Check sheet for the modelled part. Datum: model origin and axes. Units: mm. A direction names the side the tool comes from. Round coordinates to 2 decimals unless told otherwise and drop trailing zeros. Write each loop counter-clockwise with the first axis right and the second up, starting at its lowest first coordinate (ties: lowest second). Pieces come first, ordered by that corner, then holes.
Item 1: Go/stop test with flat-tipped pins: pin 1 Ø0.5 at (x, z) = (5, 3.5) entering from -Y; pin 2 Ø0.8 at (x, z) = (6, 3.5) entering from +Y; pin 3 Ø1.1 at (x, y) = (8.5, -21.5) entering from +Z. Record where each tip stops, or that it passes through.
Item 2: Cross-section at D-D on x = 6.35. Enter the section's corners in (y, z) (3 decimals).
Item 3: Cross-section at B-B on x = 11.5. Enter the section's corners in (y, z) (3 decimals), plus the area to 3 significant figures.
Item 4: Tool access check on faces 1 (the flat face through (6, -20.32, 3)), 2 (the flat face through (6, -6, 2.54)), 3 (the cylindrical face through (6.439, -25.038, 0.382)). Record the directions out of +Z, -Z, +X, -X, +Y, -Y that give a thin tool (end or side, any length) a straight path to the whole face; none if there is none.
Item 5: Cross-section at A-A on y = -6.35. Enter the section's corners in (x, z), plus the area to 3 significant figures.
Item 6: Release check for a two-part mould opening along Y. For faces 4 (the flat face through (6, -21, 1.778)), 5 (the flat face through (6, -23, 3.81)), 6 (the flat face through (6, -25.4, 2)) record: +Y half, -Y half, draft (parallel to the pull), parting line (faces both ways), or undercut.
Item 7: Cross-section at C-C on z = 0.5. Enter the section's corners in (x, y).
Item 8: Material ranges on line 1 (X direction, y = -6.35, z = 3.2); line 2 (Y direction, x = 6, z = 3.05); line 3 (Y direction, x = 6.35, z = 3.25), recorded low to high.
from build123d import *

# Parameters (mm, degrees)
F0_W        = 12.7
F0_H        = 25.4
F1_DEPTH    = 3.81
F2_R        = 4.826
F3_DEPTH    = 1.27
F4_W        = 2.032
F4_H        = 2.032
F5_DEPTH    = 25.4
F6_R        = 0.508
F7_T1_DEPTH = 22.225
F8_R        = 1.27


# Not quite as in the source:
# - a fillet or chamfer that OpenCascade refuses, or shapes differently, is made with other operations: its cross-section is extruded or revolved along the edge and cut away or added


with BuildPart() as f1:
    # F0 (on Top) → F1 (new body)
    with BuildSketch(Plane.XY):
        with Locations((6.35, -12.7)):
            Rectangle(F0_W, F0_H)
    extrude(amount=F1_DEPTH)

    # F2 (on face) → F3 (cut)
    with BuildSketch(Plane.XY.offset(3.81)):
        with Locations((6.35, -6.35)):
            Circle(F2_R)
    extrude(amount=-F3_DEPTH, mode=Mode.SUBTRACT)

    # F4 (on face) → F5 (cut)
    with BuildSketch(Plane.YZ.offset(12.7)):
        with Locations((-21.336, 2.794)):
            Rectangle(F4_W, F4_H)
    extrude(amount=-F5_DEPTH, mode=Mode.SUBTRACT)

    # F6
    f6_edges = [f1.edges().sort_by_distance(p)[0] for p in [
        (6.35, -20.32, 1.778),
        (6.35, -22.352, 1.778),
    ]]
    fillet(f6_edges, radius=F6_R)

    # F7: fillet of radius 1.905 on 2 edges, made by hand

    # F7_s2 → F7_t1 (cut)
    with BuildSketch(Plane.YZ.offset(-4.7625)):
        with BuildLine():
            ThreePointArc((0, 1.905), (-0.5579615818, 0.5579615818), (-1.905, 0))
            Line((-1.905, 0), (0, 0))
            Line((0, 0), (0, 1.905))
        make_face()
        with BuildLine():
            ThreePointArc((-1.905, 3.81), (-0.5579615818, 3.2520384182), (0, 1.905))
            Line((0, 1.905), (0, 3.81))
            Line((0, 3.81), (-1.905, 3.81))
        make_face()
    extrude(amount=F7_T1_DEPTH, mode=Mode.SUBTRACT)

    # F8
    f8_edges = [f1.edges().sort_by_distance(p)[0] for p in [
        (6.35, -25.4, 3.81),
        (6.35, -25.4, 0),
    ]]
    fillet(f8_edges, radius=F8_R)


solid = f1.part
Response values:
1. pin 1: stops at y = -25.18
1. pin 2: stops at y = -0.42
1. pin 3: stops at z = 1.82
2. outline: (-25.4, 1.27) arc R1.27 ccw to (-24.13, 0) - (-1.905, 0) arc R1.905 ccw to (-1.524, 3.772) - (-1.524, 2.54) - (-11.176, 2.54) - (-11.176, 3.81) - (-20.32, 3.81) - (-20.32, 2.286) arc R0.508 cw to (-20.828, 1.778) - (-21.844, 1.778) arc R0.508 cw to (-22.352, 2.286) - (-22.352, 3.81) - (-24.13, 3.81) arc R1.27 ccw to (-25.4, 2.54) - close
3. outline: (-25.4, 1.27) arc R1.27 ccw to (-24.13, 0) - (-1.905, 0) arc R1.905 ccw to (-1.905, 3.81) - (-20.32, 3.81) - (-20.32, 2.286) arc R0.508 cw to (-20.828, 1.778) - (-21.844, 1.778) arc R0.508 cw to (-22.352, 2.286) - (-22.352, 3.81) - (-24.13, 3.81) arc R1.27 ccw to (-25.4, 2.54) - close
3. area: 90.5 mm2
4. face 1: +Z, +X, -X
4. face 2: +Z
4. face 3: -Z, +X, -X, -Y
5. outline: (0, 0) - (12.7, 0) - (12.7, 3.81) - (11.18, 3.81) - (11.18, 2.54) - (1.52, 2.54) - (1.52, 3.81) - (0, 3.81) - close
5. area: 36.1 mm2
6. face 4: undercut
6. face 5: draft
6. face 6: -Y half
7. outline: (0, -25.14) - (12.7, -25.14) - (12.7, -0.62) - (0, -0.62) - close
8. line 1: x = 0 to 1.52, 11.18 to 12.7
8. line 2: y = -25.29 to -22.35, -20.32 to -11.16, -1.54 to -0.38
8. line 3: y = -25.18 to -22.35, -20.32 to -11.18, -1.52 to -0.56
